Read the model definition and answer for the solid it produces. Units are mm, in the model's axes. A direction names the side the tool comes from. Coordinates: 2 decimals unless noted, no trailing zeros. Loops run counter-clockwise (first coordinate to the right, second up) from the corner with the lowest first, then second, coordinate; pieces in that order, holes last.
Q1. Which of the six approach directions +Z, -Z, +X, -X, +Y, -Y give full straight-line access (tool end or side, diameter ignored) to faces 1 (the face through (-72.618, 21, -3)), 2 (the face through (29.998, 85, -3)), 3 (the face through (-59.41, -116, -3))?
Q2. Section D-D (z = -1.7) is taken. Count the separate pieces of the cut face and the enclosed holes in it, then the cut area to 3 significant figures.
Q3. Section B-B (y = 15.5) is taken. Give the vertices of the cut face in (x, z).
Q4. Straight lines are drawn through the part: line 1 (X direction, y = -34.5, z = -2); line 2 (Y direction, x = -65, z = -2.4); line 3 (X direction, y = 126.5, z = -4.6). For each, find the intervals that lie inside material, in ascending order.
Q5. Section C-C (x = -16.5) is taken. Give the vertices of the cut face in (y, z).
Q6. Section A-A (x = -53.5) is taken. Give the vertices of the cut face in (y, z).
Q7. The mould has two halves that part along Y. Classify faces 4 (the face through (-76, -93.528, -3)), 5 (the face through (35.84, -103, -3)), 6 (the face through (-21, -113.086, -3)), 7 (the face through (33, 8.072, -3)): pulls with the +Y half, pulls with the -Y half, needs draft (parallel to the pull), parting line crosses it, or undercut.
Q8. Flat-ended cylindrical pins translate along their axes: P1, Ø1.8, axis at x = -64.5, z = -4, coming from the -Y side; P2, Ø1.8, axis at y = -85, z = -3.5, coming from the -X side. Find the tip coordinate at first contact, or state that the pin passes through.
from build123d import *

# Parameters (mm, degrees)
F0_W     = 114.3
F0_H     = 262.89
F1_DEPTH = 5.842
F2_W     = 25.4
F2_H     = 5.842
F2_W_2   = 19.05
F2_W_3   = 5.842
F2_H_2   = 25.4
F3_DEPTH = 5.842
F4_R     = 4.7625
F4_R_2   = 9.525
F5_DEPTH = 5.842


# Not quite as in the source:
# - a feature names something its author has since deleted; it is built from what else it names


with BuildPart() as f1:
    # F0 (on Top) → F1 (new body)
    with BuildSketch(Plane.XY):
        with Locations((-21.309719372, 12.5171500933)):
            Rectangle(F0_W, F0_H)
    extrude(amount=-F1_DEPTH)

    # F2 (on face) → F3 (cut, through all)
    with BuildSketch(Plane.XY):
        with Locations((-21.309719372, -116.0068499067)):
            Rectangle(F2_W, F2_H)
        with Locations((-68.934719372, -116.0068499067)):
            Rectangle(F2_W_2, F2_H)
        with Locations((26.315280628, -116.0068499067)):
            Rectangle(F2_W_2, F2_H)
        with Locations((-75.538719372, -80.8278499067)):
            Rectangle(F2_W_3, F2_H_2)
        with Locations((32.919280628, -80.8278499067)):
            Rectangle(F2_W_3, F2_H_2)
        with Locations((32.919280628, -30.0278499067)):
            Rectangle(F2_W_3, F2_H_2)
        with Locations((-75.538719372, -30.0278499067)):
            Rectangle(F2_W_3, F2_H_2)
        with Locations((-75.538719372, 20.7721500933)):
            Rectangle(F2_W_3, F2_H_2)
        with Locations((32.919280628, 20.7721500933)):
            Rectangle(F2_W_3, F2_H_2)
        with Locations((-75.538719372, 71.5721500933)):
            Rectangle(F2_W_3, F2_H_2)
        with Locations((32.919280628, 71.5721500933)):
            Rectangle(F2_W_3, F2_H_2)
        with Locations((-75.538719372, 96.9721500933)):
            Rectangle(F2_W_3, F2_H_2)
        with Locations((32.919280628, 96.9721500933)):
            Rectangle(F2_W_3, F2_H_2)
    extrude(amount=-F3_DEPTH, mode=Mode.SUBTRACT)

    # F4 (on face) → F5 (cut, through all)
    with BuildSketch(Plane.XY):
        with Locations((-34.009719372, 134.4371500933)):
            Circle(F4_R)
        with Locations((-8.609719372, 134.4371500933)):
            Circle(F4_R)
        with Locations((-53.059719372, 131.2621500933)):
            Circle(F4_R_2)
        with Locations((10.440280628, 131.2621500933)):
            Circle(F4_R_2)
    extrude(amount=-F5_DEPTH, mode=Mode.SUBTRACT)


solid = f1.part
Numbers:
1. face 1: +Z, -Z, -X
1. face 2: +Z, -Z, +X
1. face 3: +Z, -Z, -X, -Y
2. separate pieces: 1
2. enclosed holes: 4
2. area: 27,500 mm2
3. outline: (-72.62, -5.84) - (30, -5.84) - (30, 0) - (-72.62, 0) - close
4. line 1: x = -72.62 to 30
4. line 2: y = -113.09 to 143.96
4. line 3: x = -78.46 to -61.31, -44.81 to 2.19, 18.69 to 35.84
5. outline: (-113.09, -5.84) - (143.96, -5.84) - (143.96, 0) - (-113.09, 0) - close
6. outline: (-118.93, -5.84) - (121.75, -5.84) - (121.75, 0) - (-118.93, 0) - close; (140.78, -5.84) - (143.96, -5.84) - (143.96, 0) - (140.78, 0) - close
7. face 4: undercut
7. face 5: needs draft
7. face 6: pulls with the -Y half
7. face 7: undercut
8. P1: stops at y = -113.09
8. P2: stops at x = -72.62
